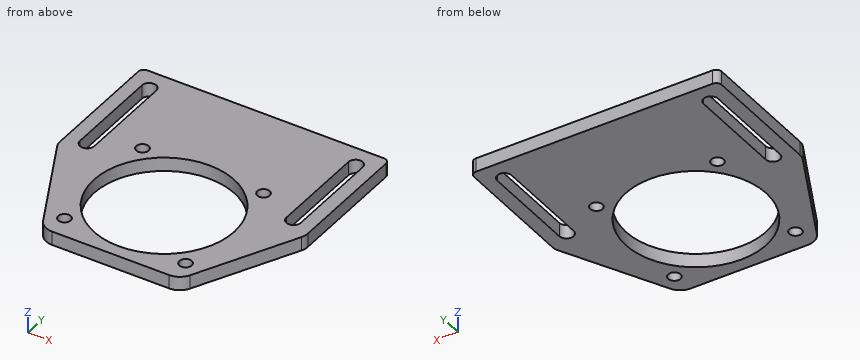
Autodesk Inventor part; units mm, degrees
ref_plane "YZ Plane" through (0, 0, 0) normal (1, 0, 0) x (0, 1, 0)
ref_plane "XZ Plane" through (0, 0, 0) normal (0, 1, 0) x (-1, 0, 0)
ref_plane "XY Plane" through (0, 0, 0) normal (0, 0, 1) x (1, 0, 0)
sketch "Sketch1" plane through (0, 0, 0) normal (0, 0, 1) x (1, 0, 0)
  line L0 (-45, 43.75) -> (45, 43.75)
  line L1 (45, 43.75) -> (45, -3.75)
  line L2 (45, -3.75) -> (25, -43.75)
  line L3 (25, -43.75) -> (-25, -43.75)
  line L4 (-25, -43.75) -> (-45, -3.75)
  line L5 (-45, -3.75) -> (-45, 43.75)
  line L6 (0, 53.6312) -> (0, 0)
  line L7 (0, 0) -> (107.3954, 0)
  line L8 (-37.5, 36.25) -> (-37.5, 1.25) construction
  line L9 (-40.1, 36.25) -> (-40.1, 1.25)
  line L10 (-34.9, 1.25) -> (-34.9, 36.25)
  arc A0 (-34.9, 36.25) -> (-40.1, 36.25) centre (-37.5, 36.25) ccw
  arc A1 (-40.1, 1.25) -> (-34.9, 1.25) centre (-37.5, 1.25) ccw
  line L11 (37.5, 36.25) -> (37.5, 1.25) construction
  line L12 (34.9, 36.25) -> (34.9, 1.25)
  line L13 (40.1, 1.25) -> (40.1, 36.25)
  arc A2 (40.1, 36.25) -> (34.9, 36.25) centre (37.5, 36.25) ccw
  arc A3 (34.9, 1.25) -> (40.1, 1.25) centre (37.5, 1.25) ccw
  line L14 (-37.5, 36.25) -> (167.5, 36.25) construction
  point P0 (-37.5, 18.75)
  point P1 (37.5, 18.75)
  dimension "d1" = 87.5
  dimension "d2" = 47.5
  dimension "d3" = 2.6
  dimension "d4" = 35
  dimension "d5" = 7.5
  dimension "d6" = 7.5
  dimension "d7" = 75
  dimension "d9" = 20
  dimension "d40" = 7.5
  dimension "d41" = 5.2
  dimension "d42" = 5.2
  dimension "d45" = 42.5
extrude "Extrusion1" add sketch "Sketch1" along normal blind 5 contours L0 L6 L7 A3 L1 L2 L3 L4 L5 | L0 L1 L7 A3 L13 A2 L12 L6
fillet "Fillet1" radius 2 2 edges at (-45, 43.75, 2.5) (45, 43.75, 2.5)
sketch "Sketch2" plane through (0, 0, 5) normal (0, 0, 1) x (1, 0, 0)
  line L0 (0.1, -13.75) -> (0.1, 26.1696) construction
  line L1 (-34.9, 36.25) -> (-34.9, 1.25)
  line L2 (-25, -43.75) -> (25, -43.75)
  point P0 (0, 0)
  point P1 (-23.7639, -52.5)
  point P2 (23.7639, -52.5)
  dimension "d23" = 35
  dimension "d24" = 30
hole "Hole1" at (0.1, -13.75, 5) direction (0, 0, -1) diameter 51 end through all
sketch "Sketch3" plane through (0, 0, 5) normal (0, 0, 1) x (1, 0, 0)
  circle A0 centre (0.1, -13.75) radius 25.5
  point P0 (0, 0)
  point P1 (-21.9, 8.25)
  dimension "d32" = 22
  dimension "d33" = 22
hole "Hole2" at (-21.9, 8.25, 5) direction (0, 0, -1) diameter 4.5 end through all
pattern_linear "Rectangular Pattern2" count 2 spacing 44 along (1, 0, 0) count 2 spacing 44 along (0, -1, 0) of "Hole2"
fillet "Rundung2" radius 6 4 edges at (45, -3.75, 2.5) (25, -43.75, 2.5) (-25, -43.75, 2.5) (-45, -3.75, 2.5)
equation "\"d6\" = d5"
equation "\"d36\" = 2 * d32"
equation "\"d39\" = 2 * d32"
properties part number "103.006.01_Dosiereinheit_Rahmenaufnahme"
Could you check a few things on this model? Use its own coordinates, in mm. Give positions to 0.01 mm unless a question says otherwise; leave off trailing zeros. Loops run counter-clockwise (first coordinate to the right, second up) from the corner with the lowest first, then second, coordinate; pieces in that order, holes last. Notation, with made-up numbers: (43, 57.5) -> (47, 57.5) arc R17 ccw to (47, 67.5) -> close; hole circle Ø1 at (-28.5, 88). An arc over 180 degrees is marked (long way). Put each result on its own line as item: value.
(1) Imagine slicing it at D-D on z = 2.8. Write out the boundary of the cut face in (x, y).
Computed:
outline: (-45, -2.33) arc R6 ccw to (-44.37, -5.02) -> (-26.66, -40.43) arc R6 ccw to (-21.29, -43.75) -> (21.29, -43.75) arc R6 ccw to (26.66, -40.43) -> (44.37, -5.02) arc R6 ccw to (45, -2.33) -> (45, 41.75) arc R2 ccw to (43, 43.75) -> (-43, 43.75) arc R2 ccw to (-45, 41.75) -> close; hole (-40.1, 1.25) arc R2.6 ccw to (-34.9, 1.25) -> (-34.9, 36.25) arc R2.6 ccw to (-40.1, 36.25) -> close; hole circle Ø51 at (0.1, -13.75); hole circle Ø4.5 at (-21.9, -35.75); hole circle Ø4.5 at (-21.9, 8.25); hole circle Ø4.5 at (22.1, -35.75); hole circle Ø4.5 at (22.1, 8.25); hole (34.9, 1.25) arc R2.6 ccw to (40.1, 1.25) -> (40.1, 36.25) arc R2.6 ccw to (34.9, 36.25) -> close
(2) I'm going to push flat-ended pins straight in: pin 1 Ø2.5 at (x, y) = (-21.9, -35.75) entering from +Z; pin 2 Ø1.5 at (y, z) = (-11.5, 1.5) entering from -X. Where does each tip first touch, or does it pass through?
Computed:
pin 1: through
pin 2: x = -41.5
(3) Please list where these lines run through material, in increasing order: probe 1 along Y at (x, z) = (-16, 3.85); probe 2 along Y at (x, z) = (-21.9, 2.9); probe 3 along Y at (x, z) = (0.5, 2.95). Write a range as [from, to].
Computed:
probe 1: [-43.75, -33.52], [6.02, 43.75]
probe 2: [-43.72, -38], [-33.5, -26.64], [-0.86, 6], [10.5, 43.75]
probe 3: [-43.75, -39.25], [11.75, 43.75]
(4) Imagine slicing it at B-B on y = 28. Write out the boundary of the cut face in (x, z), plus the area to 3 significant figures.
Computed:
outline: (-45, 0) -> (-40.1, 0) -> (-40.1, 5) -> (-45, 5) -> close; (-34.9, 0) -> (34.9, 0) -> (34.9, 5) -> (-34.9, 5) -> close; (40.1, 0) -> (45, 0) -> (45, 5) -> (40.1, 5) -> close
area: 398 mm^2
(5) Imagine slicing it at A-A on x = -37.5. Write out the boundary of the cut face in (y, z), plus the area to 4 significant figures.
Computed:
outline: (-18.75, 0) -> (-1.35, 0) -> (-1.35, 5) -> (-18.75, 5) -> close; (38.85, 0) -> (43.75, 0) -> (43.75, 5) -> (38.85, 5) -> close
area: 111.5 mm^2
(6) Imagine slicing it at C-C on y = -13.75. Write out the boundary of the cut face in (x, z), plus the area to 3 significant figures.
Computed:
outline: (-40, 0) -> (-25.4, 0) -> (-25.4, 5) -> (-40, 5) -> close; (25.6, 0) -> (40, 0) -> (40, 5) -> (25.6, 5) -> close
area: 145 mm^2
